Part print with two shaded views. Sizes in mm from the minimum x, y, z corner. A direction names the side the tool comes from. Give positions to 0.01 mm unless a question says otherwise; leave off trailing zeros. Write each loop counter-clockwise with the first axis right and the second up, starting at its lowest first coordinate (ties: lowest second). Pieces come first, ordered by that corner, then holes. Notation, with made-up numbers: M -16.75,-38 L 12.25,-38 A24 cw 12.25,-8 Z; hole C -19,56 d7. An arc over 180 degrees is marked long. One line per item, written item: value. Start each with the question number.
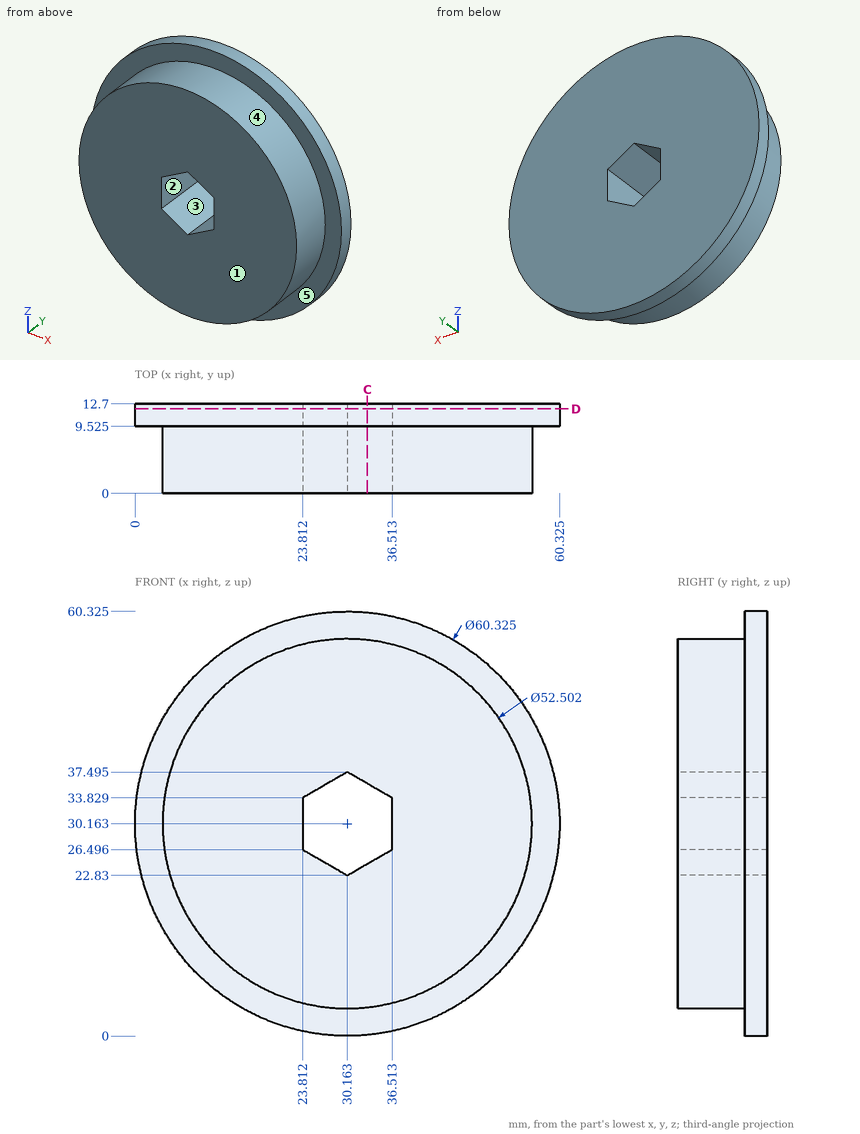
1) Drop flat-ended pins along their axis: P1, Ø2, axis at x = 54, y = 2.5, coming from the +Z side (1 decimal); P2, Ø6, axis at y = 11, z = 48.5, coming from the +X side (1 decimal); P3, Ø3, axis at x = 22.5, y = 3.5, coming from the +Z side. Give the stop position or say it passes through.
2) Mould opens along Z. For the marked faces 3, 4 and 5 say: released by +Z, released by -Z, zero draft, split by the parting line, or undercut.
3) Band-saw the part on C-C (x = 33). List the corners of the cut face in (y, z) (1 decimal).
4) Probe line 1 along X through (y, z) = (8, 33.5) (1 decimal); line 2 along Y through (x, z) = (15, 6) (1 decimal); line 3 along X through (y, z) = (4, 11.5) (1 decimal). List the from-to ranges inside material, lowest first. Write a range as from..to.
5) Tool access for the marked faces 1 and 2: list every direction of +Z, -Z, +X, -X, +Y, -Y with a clear straight run to the whole face (end or side of a thin tool).
6) Band-saw the part on D-D (y = 12). List the corners of the cut face in (x, z) (1 decimal).
Model answer:
1. P1: stops at z = 43.1
1. P2: stops at x = 56.1
1. P3: stops at z = 55.68
2. face 3: undercut
2. face 4: split by the parting line
2. face 5: zero draft
3. outline: M 0,4.1 L 9.5,4.1 L 9.5,0.1 L 12.7,0.1 L 12.7,24.5 L 0,24.5 Z; M 0,35.9 L 12.7,35.9 L 12.7,60.2 L 9.5,60.2 L 9.5,56.3 L 0,56.3 Z
4. line 1: x = 4.1..23.8, 36.5..56.2
4. line 2: y = 9.5..12.7
4. line 3: x = 11.7..48.6
5. face 1: +Z, -Z, +X, -X, -Y
5. face 2: +Y, -Y
6. outline: C 30.2,30.2 d60.3; hole M 23.8,26.5 L 30.2,22.8 L 36.5,26.5 L 36.5,33.8 L 30.2,37.5 L 23.8,33.8 Z
